Answer from the drawing. Dimensions are ordinates in mm from the lowest x, y and z of the part. Round coordinates to 2 decimals unless told otherwise and drop trailing zeros. Write each loop counter-clockwise with the first axis right and the second up, starting at its lowest first coordinate (ties: lowest second). Pieces come first, ordered by that corner, then holes. Notation, with made-up numbers: (-37.5, -8.75) - (-26.5, -8.75) arc R27 ccw to (-26.5, 26.25) - close; hole circle Ø9 at (11, -17). An arc over 180 degrees is marked (long way). One line per item, written item: value. Start each with the question number.
(1) A cutting plane is placed at A-A, the plane y = 10. Determine the outline of the cut face in (x, z), plus the area to 3 significant figures.
(2) A flat-ended cylindrical pin translates along its axis: pin 1 Ø3 at (x, z) = (1.5, 112) entering from -Y. Find the tip coordinate at first contact, or state that the pin passes through.
(3) Find the intervals of material crossed by L1, parallel to Z at x = 3.4, y = 15.5; L2, parallel to Y at x = 2.2, z = 40; L3, parallel to Z at x = 4.2, y = 10.25, in increasing order.
(4) A cutting plane is placed at B-B, the plane z = 40. Determine the outline of the cut face in (x, y).
(5) A cutting plane is placed at C-C, the plane x = 1.95. Determine the outline of the cut face in (y, z).
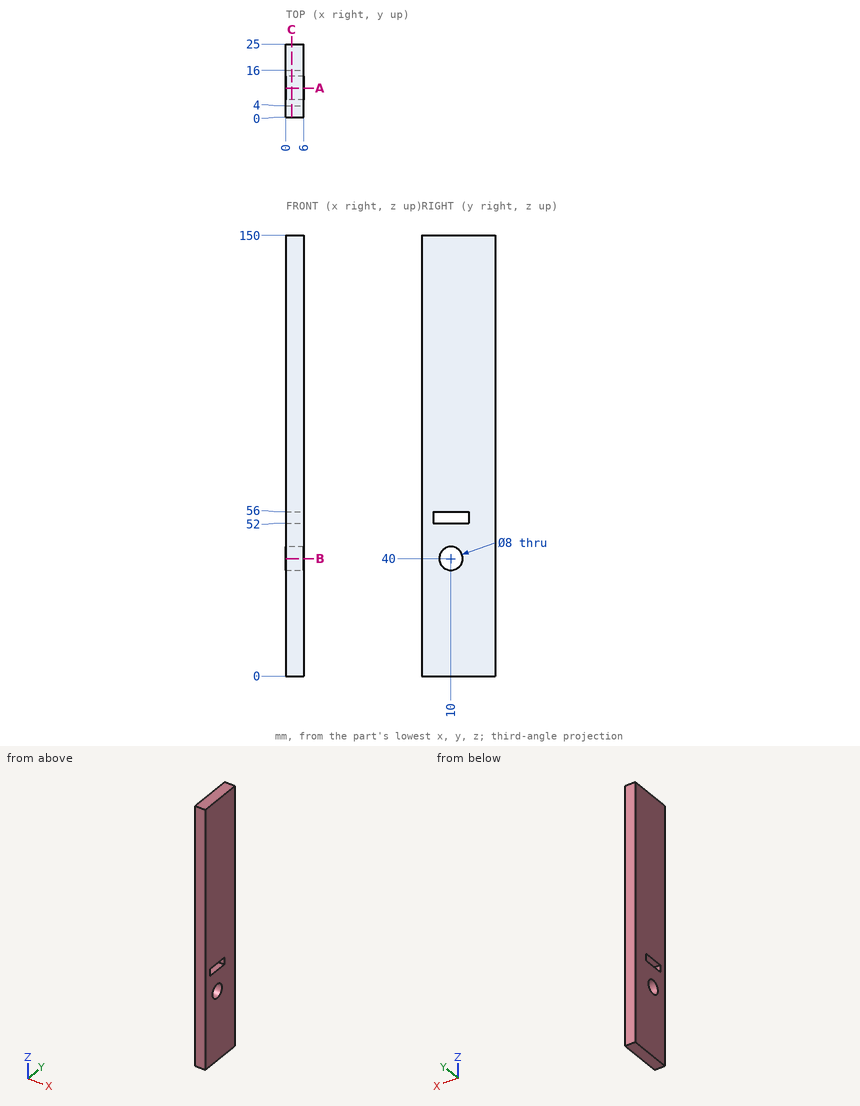
Here are the results:
1. outline: (0, 0) - (6, 0) - (6, 36) - (0, 36) - close; (0, 44) - (6, 44) - (6, 52) - (0, 52) - close; (0, 56) - (6, 56) - (6, 150) - (0, 150) - close
1. area: 828 mm²
2. pin 1: y = 0
3. L1: 0 to 52, 56 to 150
3. L2: 0 to 6, 14 to 25
3. L3: 0 to 36.01, 43.99 to 52, 56 to 150
4. outline: (0, 0) - (6, 0) - (6, 6) - (0, 6) - close; (0, 14) - (6, 14) - (6, 25) - (0, 25) - close
5. outline: (0, 0) - (25, 0) - (25, 150) - (0, 150) - close; hole (4, 52) - (16, 52) - (16, 56) - (4, 56) - close; hole circle Ø8 at (10, 40)
